Verification items for the finished model (mm, model axes). Face numbers are marked on the shaded views. A direction names the side the tool comes from. Coordinates: 2 decimals unless noted, no trailing zeros. Write each loop counter-clockwise with the first axis right and the second up, starting at its lowest first coordinate (ties: lowest second). Pieces come first, ordered by that corner, then holes. Notation, with made-up numbers: (12, 58.25) - (29, 58.25) arc R32 ccw to (29, 91.25) - close; hole circle Ø11 at (-35.75, 38.5). An arc over 180 degrees is marked (long way). Use one line per item in the form item = value. Start each with the question number.
(1) Sectioned sample at A-A (z = 21). Record the cut outline in (x, y).
(2) Gauge pin test, flat ends, axial feed: pin 1 Ø2 at (x, y) = (31.5, 35.5) entering from +Z; pin 2 Ø5 at (x, y) = (48.5, 24) entering from +Z. Record the tip position at first contact, or that the pin passes through.
(3) Sectioned sample at C-C (x = 22.5). Record the cut outline in (y, z).
(4) Sectioned sample at B-B (y = 24). Record the cut outline in (x, z).
(5) Sectioned sample at D-D (z = 33.5). Record the cut outline in (x, y).
(6) Tool access check on the marked faces 1, 2 and 3. Record the directions out of +Z, -Z, +X, -X, +Y, -Y that give a thin tool (end or side, any length) a straight path to the whole face; none if there is none.
(7) Material ranges on line 1 (X direction, y = 32, z = 9); line 2 (X direction, y = 15.5, z = 47), recorded low to high. Write a range as [from, to].
Solid Edge part; units mm, degrees
sketch "Sketch1" plane through (0, 0, 0) normal (1, 0, 0) x (0, 1, 0)
  line L0 (0, 0) -> (43.8289, 0)
sketch "Sketch2" plane through (0, 0, 0) normal (0, -1, 0) x (1, 0, 0)
  line L0 (0, 50.8) -> (0, 0)
  line L1 (0, 0) -> (50.8, 0)
  line L2 (50.8, 27.381) -> (50.8, 0)
  line L3 (44.45, 27.381) -> (50.8, 27.381)
  line L4 (44.45, 6.35) -> (44.45, 27.381)
  line L5 (44.45, 6.35) -> (6.35, 6.35)
  line L6 (6.35, 6.35) -> (6.35, 50.8)
  line L7 (6.35, 50.8) -> (0, 50.8)
sweep "SweptProtrusion_1" add profiles "Sketch2" path "Sketch1"
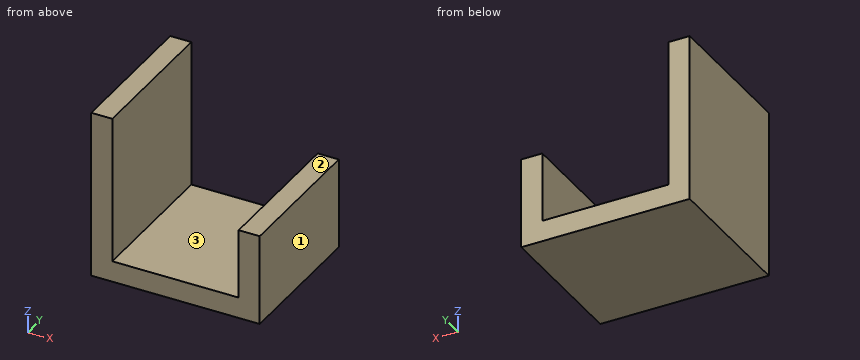
Answers below:
q1.outline = (0, 0) - (6.35, 0) - (6.35, 43.83) - (0, 43.83) - close; (44.45, 0) - (50.8, 0) - (50.8, 43.83) - (44.45, 43.83) - close
q2.pin_1 = 6.35
q2.pin_2 = 27.38
q3.outline = (0, 0) - (43.83, 0) - (43.83, 6.35) - (0, 6.35) - close
q4.outline = (0, 0) - (50.8, 0) - (50.8, 27.38) - (44.45, 27.38) - (44.45, 6.35) - (6.35, 6.35) - (6.35, 50.8) - (0, 50.8) - close
q5.outline = (0, 0) - (6.35, 0) - (6.35, 43.83) - (0, 43.83) - close
q6.face_1 = +Z, -Z, +X, +Y, -Y
q6.face_2 = +Z, +X, +Y, -Y
q6.face_3 = +Z, +Y, -Y
q7.line_1 = [0, 6.35], [44.45, 50.8]
q7.line_2 = [0, 6.35]
